Could you check a few things on this drawing? It's one solid part, dimensions in mm from its lowest x, y, z. A direction names the side the tool comes from. Give positions to 0.01 mm unless a question says otherwise; leave off trailing zeros. Loops run counter-clockwise (first coordinate to the right, second up) from the corner with the lowest first, then second, coordinate; pieces in that order, holes last. Notation, with made-up numbers: (-29, 51.5) -> (0, 51.5) arc R9 cw to (0, 57.5) -> close; hole circle Ø9 at (44, 70). An arc over 180 degrees is marked (long way). Use CSV: the item, a comma, the result in double quotes.
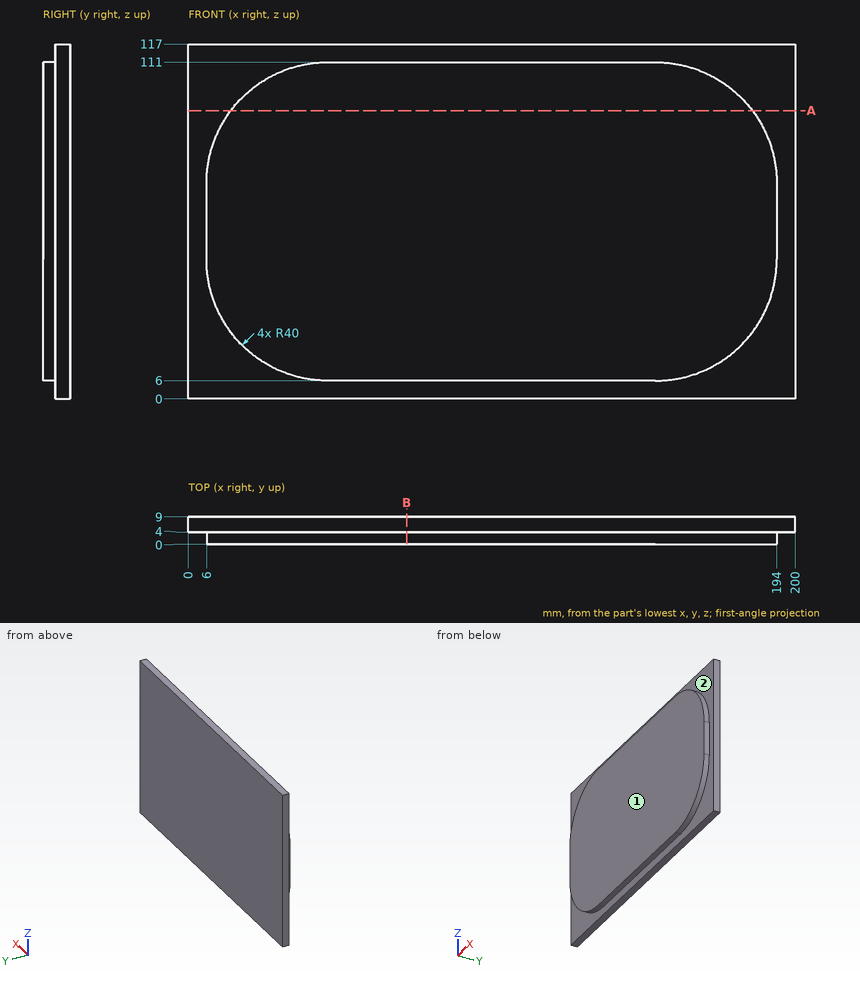
(1) Which directions (+Z, -Z, +X, -X, +Y, -Y) give clear straight access to the entire face, cutting with the end or side of a thin tool? Please do the marked faces 1 and 2.
Answer sheet:
face 1,"+Z, -Z, +X, -X, -Y"
face 2,"-Y"
(2) If we section it at A-A, the plane z = 95: Write out the boundary of the cut face in (x, y), then the cut area to 3 significant figures.
Answer sheet:
outline,"(0, 4) -> (14, 4) -> (14, 0) -> (186, 0) -> (186, 4) -> (200, 4) -> (200, 9) -> (0, 9) -> close"
area,"1,690 mm2"
(3) Will these pins go through, and if not, where does the flat tip stop? pin 1 Ø1.5 at (y, z) = (1.5, 103) entering from +X; pin 2 Ø3 at (y, z) = (2, 53) entering from +X; pin 3 Ø2 at (y, z) = (2, 60) entering from -X.
Answer sheet:
pin 1,"stops at x = 178.97"
pin 2,"stops at x = 194"
pin 3,"stops at x = 6"
(4) If we section it at B-B, the plane x = 72: Write out the boundary of the cut face in (y, z).
Answer sheet:
outline,"(0, 6) -> (4, 6) -> (4, 0) -> (9, 0) -> (9, 117) -> (4, 117) -> (4, 111) -> (0, 111) -> close"
(5) If I drill on L1, parallel to Z at x = 56, y = 2.75; L2, parallel to X at y = 2.25, z = 61.5; L3, parallel to X at y = 1.75, z = 80, over which ranges is the centre line in solid material (lowest first)? Write a range as from..to.
Answer sheet:
L1,"z = 6..111"
L2,"x = 6..194"
L3,"x = 7.03..192.97"
